Source: CAD feature listing. Evaluate the final solid. Frame: model axes, mm. Face numbers are marked on the shaded views. A direction names the side the tool comes from. Give positions to 0.01 mm unless a question says otherwise; leave off trailing zeros. Loops run counter-clockwise (first coordinate to the right, second up) from the corner with the lowest first, then second, coordinate; pieces in that order, holes last. Notation, with made-up numbers: (-31.75, -34.5) -> (11.25, -34.5) arc R26 ccw to (11.25, -7.5) -> close; hole circle Ø5 at (-13.75, 84). An arc over 180 degrees is marked (long way). Return JSON: item names as keys, results as strings. Group by question number.
(1) Cut plane C-C on y = -65. Return loops of the section in (x, z).
(2) Cut plane B-B on x = 18. Return loops of the section in (y, z), then the cut area to 3 significant figures.
(3) Cut plane D-D on z = 15. Return loops of the section in (x, y), then the cut area to 3 significant figures.
(4) Draft query along Y for the marked faces 5, 6 and 7. Return one class per face: released by +Y, released by -Y, zero draft, split by the parting line, or undercut.
(5) Ray query, line 1 (X direction, y = 7, z = 31); line 2 (Z direction, x = 5.5, y = 4); line 3 (X direction, y = -65, z = 8.5). Return the intervals inside material, ascending. Write a range as from..to.
(6) Pin query (flat end, axial travel): pin 1 (1.5 mm diameter, centred on x = 53.5, z = 45.5, fed in from +Y); pin 2 (14.5 mm diameter, centred on y = -22, z = 6, fed in from +X); pin 3 (8 mm diameter, centred on x = 70, y = -52, fed in from +Z). Return the tip coordinate at first contact, or that it passes through.
(7) Access query for the marked faces 1, 2, 3 and 4. Directions: +Z, -Z, +X, -X, +Y, -Y. A direction counts if a zero-diameter tool reaches every point of the face in a straight line with its end or side. Return the directions, or none.
(8) Cut plane A-A on z = 31.5. Return loops of the section in (x, y), then the cut area to 3 significant figures.
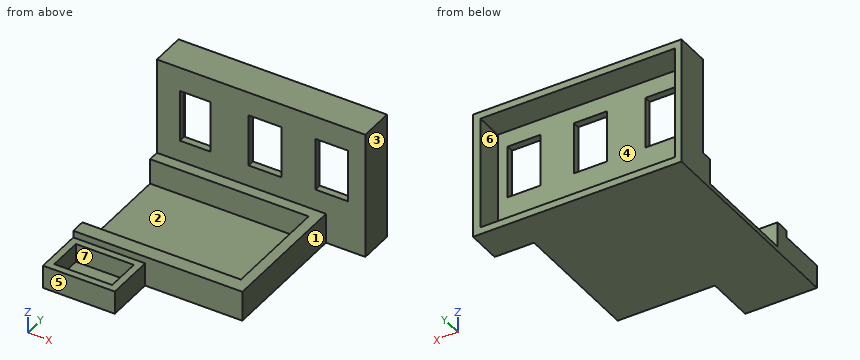
```python
from build123d import *

# Parameters (mm, degrees)
F0_W      = 73
F0_H      = 58
F1_DEPTH  = 13
F2_W      = 63.252263
F2_H      = 46.978496
F3_DEPTH  = 11
F4_W      = 5.207941
F4_H      = 46.978496
F5_DEPTH  = 11
F6_W      = 90
F6_H      = 15
F7_DEPTH  = 55
F8_W      = 84.081179
F8_H      = 48.908066
F9_DEPTH  = 12
F10_W     = 31
F10_H     = 21
F11_DEPTH = 10
F12_W     = 25
F12_H     = 15
F13_DEPTH = 8
F14_W     = 13.124006
F14_H     = 22.36615
F14_W_2   = 14.341504
F14_H_2   = 22.587417
F14_W_3   = 14.118343
F14_H_3   = 22.820918
F15_DEPTH = 25


with BuildPart() as f1:
    # F0 (on Top) → F1 (new body)
    with BuildSketch(Plane.XY):
        with Locations((36.5, -29)):
            Rectangle(F0_W, F0_H)
    extrude(amount=F1_DEPTH)

    # F2 (on face) → F3 (cut)
    with BuildSketch(Plane.XY.offset(13)):
        with Locations((36.834072, -28.219316)):
            Rectangle(F2_W, F2_H)
    extrude(amount=-F3_DEPTH, mode=Mode.SUBTRACT)

    # F4 (on face) → F5 (cut)
    with BuildSketch(Plane.XY.offset(13)):
        with Locations((2.60397, -28.219316)):
            Rectangle(F4_W, F4_H)
    extrude(amount=-F5_DEPTH, mode=Mode.SUBTRACT)

    # F6 (on Top) → F7 (join)
    with BuildSketch(Plane.XY):
        with Locations((45, 7.5)):
            Rectangle(F6_W, F6_H)
    extrude(amount=F7_DEPTH)

    # F8 (on face) → F9 (cut)
    with BuildSketch(Plane(origin=(0, 15, 0), x_dir=(-1, 0, 0), z_dir=(0, 1, 0))):
        with Locations((-44.739444, 27.506275)):
            Rectangle(F8_W, F8_H)
    extrude(amount=-F9_DEPTH, mode=Mode.SUBTRACT)

    # F10 (on Top) → F11 (join)
    with BuildSketch(Plane.XY):
        with Locations((15.5, -68.5)):
            Rectangle(F10_W, F10_H)
    extrude(amount=F11_DEPTH)

    # F12 (on face) → F13 (cut)
    with BuildSketch(Plane.XY.offset(10)):
        with Locations((15.5, -68.5)):
            Rectangle(F12_W, F12_H)
    extrude(amount=-F13_DEPTH, mode=Mode.SUBTRACT)

    # F14 (on face) → F15 (cut)
    with BuildSketch(Plane.XZ):
        with Locations((16.504721, 33.388489)):
            Rectangle(F14_W, F14_H)
        with Locations((46.720475, 33.499122)):
            Rectangle(F14_W_2, F14_H_2)
        with Locations((75.470149, 33.615873)):
            Rectangle(F14_W_3, F14_H_3)
    extrude(amount=-F15_DEPTH, mode=Mode.SUBTRACT)


solid = f1.part
```
Answers:
{
 "1": {"outline": "(0, 0) -> (31, 0) -> (31, 10) -> (28, 10) -> (28, 2) -> (3, 2) -> (3, 10) -> (0, 10) -> close"},
 "2": {"outline": "(-79, 0) -> (15, 0) -> (15, 3.05) -> (3, 3.05) -> (3, 22.21) -> (0, 22.21) -> (0, 13) -> (-4.73, 13) -> (-4.73, 2) -> (-51.71, 2) -> (-51.71, 13) -> (-58, 13) -> (-58, 10) -> (-61, 10) -> (-61, 2) -> (-76, 2) -> (-76, 10) -> (-79, 10) -> close; (0, 44.57) -> (3, 44.57) -> (3, 51.96) -> (15, 51.96) -> (15, 55) -> (0, 55) -> close", "area": "498 mm²"},
 "3": {"outline": "(0, 0) -> (90, 0) -> (90, 15) -> (86.78, 15) -> (86.78, 3) -> (2.7, 3) -> (2.7, 15) -> (0, 15) -> close", "area": "341 mm²"},
 "4": {"face 5": "released by -Y", "face 6": "zero draft", "face 7": "undercut"},
 "5": {"line 1": "0..2.7, 86.78..90", "line 2": "0..3.05, 51.96..55", "line 3": "0..3, 28..31"},
 "6": {"pin 1": "y = 3", "pin 2": "x = 73", "pin 3": "z = 13"},
 "7": {"face 1": "+Z, -Z, +X, -Y", "face 2": "+Z, -X", "face 3": "+Z, -Z, +X, +Y, -Y", "face 4": "+Y"},
 "8": {"outline": "(0, 0) -> (9.94, 0) -> (9.94, 3) -> (2.7, 3) -> (2.7, 15) -> (0, 15) -> close; (23.07, 0) -> (39.55, 0) -> (39.55, 3) -> (23.07, 3) -> close; (53.89, 0) -> (68.41, 0) -> (68.41, 3) -> (53.89, 3) -> close; (82.53, 0) -> (90, 0) -> (90, 15) -> (86.78, 15) -> (86.78, 3) -> (82.53, 3) -> close", "area": "216 mm²"}
}
